Source: CAD feature listing. Evaluate the final solid. Frame: model axes, mm. Give positions to 0.01 mm unless a question says otherwise; leave off trailing zeros. Order: outer loops, then holes, each group sorted by start corner. A loop starts at its lowest first (then second) coordinate and runs counter-clockwise, first axis right, second up.
from build123d import *

# Parameters (mm, degrees)
SKETCH1_W           = 133.35
SKETCH1_H           = 25.4
BOSS_EXTRUDE1_DEPTH = 6.35
SKETCH2_R           = 1.5875
CUT_EXTRUDE1_DEPTH  = 6.35


with BuildPart() as part:
    # Sketch1 → Boss-Extrude1 (new body)
    with BuildSketch(Plane(origin=(0, 0, 0), x_dir=(1, 0, 0), z_dir=(0, 1, 0))):
        Rectangle(SKETCH1_W, SKETCH1_H)
    extrude(amount=BOSS_EXTRUDE1_DEPTH)

    # Sketch2 → Cut-Extrude1 (cut)
    with BuildSketch(Plane(origin=(0, 6.35, 0), x_dir=(1, 0, 0), z_dir=(0, 1, 0))):
        with Locations(Location((0, 7.62, 0), (0, 0, 270))):
            Circle(SKETCH2_R)
        with Locations(Location((-12.7, 7.62, 0), (0, 0, 270))):
            Circle(SKETCH2_R)
        with Locations(Location((12.7, 7.62, 0), (0, 0, 270))):
            Circle(SKETCH2_R)
        with Locations(Location((-48.895, -7.62, 0), (0, 0, 270))):
            Circle(SKETCH2_R)
        with Locations(Location((-40.005, -7.62, 0), (0, 0, 270))):
            Circle(SKETCH2_R)
        with Locations(Location((-31.115, -7.62, 0), (0, 0, 270))):
            Circle(SKETCH2_R)
        with Locations(Location((-13.335, -7.62, 0), (0, 0, 270))):
            Circle(SKETCH2_R)
        with Locations(Location((-22.225, -7.62, 0), (0, 0, 270))):
            Circle(SKETCH2_R)
        with Locations(Location((-4.445, -7.62, 0), (0, 0, 270))):
            Circle(SKETCH2_R)
        with Locations(Location((4.445, -7.62, 0), (0, 0, 270))):
            Circle(SKETCH2_R)
        with Locations(Location((13.335, -7.62, 0), (0, 0, 270))):
            Circle(SKETCH2_R)
        with Locations(Location((22.225, -7.62, 0), (0, 0, 270))):
            Circle(SKETCH2_R)
        with Locations(Location((31.115, -7.62, 0), (0, 0, 270))):
            Circle(SKETCH2_R)
        with Locations(Location((40.005, -7.62, 0), (0, 0, 270))):
            Circle(SKETCH2_R)
        with Locations(Location((48.895, -7.62, 0), (0, 0, 270))):
            Circle(SKETCH2_R)
    extrude(amount=-CUT_EXTRUDE1_DEPTH, mode=Mode.SUBTRACT)


solid = part.part
1) Section query A-A on z = -7.62. State how many separate pieces and enclosed holes the cut face has, and give its area (3 significant figures).
Checks:
separate pieces: 4
enclosed holes: 0
area: 786 mm2
2) Pull-direction query (Z, two-part tool) for faces 1 (the face through (-1, 3, 12.7)), 2 (the face through (-66.675, 3, 0)), 3 (the face through (23.3, 3.22, 6.45)); classes: +Z half, -Z half, draft (parallel to the pull), parting line (faces both ways), or undercut.
Checks:
face 1: +Z half
face 2: draft
face 3: undercut
3) First-contact query: pin 1 Ø5 at (x, z) = (-4.445, 7.62) entering from +Y. Flat tip, straight axial feed; report the tip coordinate or a pass-through.
Checks:
pin 1: stops at y = 6.35
4) Section query B-B on x = 0. Output: boundary loops of the cut face in (y, z).
Checks:
outline: (0, -12.7) - (6.35, -12.7) - (6.35, -9.21) - (0, -9.21) - close; (0, -6.03) - (6.35, -6.03) - (6.35, 12.7) - (0, 12.7) - close
5) Ray query, L1, parallel to X at y = 2.25, z = -7.75 (3 decimals); L2, parallel to X at y = 4.25, z = -8.25 (3 decimals); L3, parallel to Z at x = -48.5, y = 1.5. Return the intervals inside material, ascending.
Checks:
L1: x = -66.675 to -14.282, -11.118 to -1.582, 1.582 to 11.118, 14.282 to 66.675
L2: x = -66.675 to -14.157, -11.243 to -1.457, 1.457 to 11.243, 14.157 to 66.675
L3: z = -12.7 to 6.08, 9.16 to 12.7
